from build123d import *

# Parameters (mm, degrees)
BOSS_EXTRUDE1_DEPTH          = 41.656
CUT_EXTRUDE1_DEPTH           = 38.481
CUT_EXTRUDE2_START           = -28.8671
SKETCH11_W                   = 16.434556017
SKETCH11_H                   = 15.968225366
CUT_EXTRUDE2_DEPTH           = 7.62
SKETCH16_W                   = 24.568216569
SKETCH16_H                   = 19.806256701
BOSS_EXTRUDE3_DEPTH          = 53.34
CUT_EXTRUDE3_START           = -24.568216569
CUT_EXTRUDE3_DEPTH           = 24.568216569
SKETCH22_W                   = 16.862412739
SKETCH22_H                   = 15.968225366
CUT_EXTRUDE4_DEPTH           = 53.34
CUT_EXTRUDE6_DEPTH           = 119.901499034
F_10_0_1935_DIAMETER_HOLE1_D = 4.9149
CUT_EXTRUDE11_REACH          = 116.77
CUT_EXTRUDE9_DEPTH           = 112.875933154
FILLET2_R                    = 2.54
SKETCH34_W                   = 28.194
SKETCH34_H                   = 38.481
BOSS_EXTRUDE4_DEPTH          = 3.302


# Read off the part's stored shape, not the designer's step: Cut-Extrude3
with BuildPart() as part:
    # Sketch1 → Boss-Extrude1 (new body)
    with BuildSketch(Plane(origin=(0, 0, 0), x_dir=(1, 0, 0), z_dir=(0, 1, 0))):
        with BuildLine():
            Line((63.017839503, -66.782093), (53.468205472, -26.506342671))
            Line((53.468205472, -26.506342671), (-35.875703335, -47.690346072))
            Line((-35.875703335, -47.690346072), (-26.326069304, -87.966096401))
            ThreePointArc((-26.326069304, -87.966096401), (21.184003401, -89.343908807), (63.017839503, -66.782093))
        make_face()
    extrude(amount=BOSS_EXTRUDE1_DEPTH)

    # Sketch2 → Cut-Extrude1 (cut)
    with BuildSketch(Plane(origin=(0, 41.656, 0), x_dir=(1, 0, 0), z_dir=(0, 1, 0))):
        Polygon((19.413866358, -81.878324539), (52.259801297, -74.090346526), (45.755169548, -46.656947141), (-3.674378893, -58.377004348), (2.830252857, -85.810403732), align=None)
    extrude(amount=-CUT_EXTRUDE1_DEPTH, mode=Mode.SUBTRACT)

    # Sketch11 → Cut-Extrude2 (cut)
    with BuildSketch(Plane(origin=(-44.671954403, 0, 10.592001701), x_dir=(0.230709787533386, 0, 0.973022607104429), z_dir=(-0.973022607104429, 0, 0.230709787533386)).offset(CUT_EXTRUDE2_START)):
        with Locations((69.159923537, 24.869161711)):
            Rectangle(SKETCH11_W, SKETCH11_H)
    extrude(amount=CUT_EXTRUDE2_DEPTH, mode=Mode.SUBTRACT)

    # Sketch16 → Boss-Extrude3 (add)
    with BuildSketch(Plane(origin=(-33.786311583, 0, 16.678693854), x_dir=(0, -1, 0), z_dir=(0.8966923373350206, 0, -0.4426543258171746))):
        with Locations((-23.482416275, -61.32247831)):
            Rectangle(SKETCH16_W, SKETCH16_H)
    extrude(amount=-BOSS_EXTRUDE3_DEPTH)

    # Cut-Extrude3 outline → Cut-Extrude3 (cut)
    with BuildSketch(Plane(origin=(0, 35.766524559, 0), x_dir=(1, 0, 0), z_dir=(0, 1, 0)).offset(CUT_EXTRUDE3_START)):
        with BuildLine():
            Line((-50.087557959, -104.157331307), (-20.43350094, -89.518534843))
            ThreePointArc((-20.43350094, -89.518534843), (-33.301223909, -85.569413503), (-45.453344654, -79.781511021))
            Line((-45.453344654, -79.781511021), (-58.854883166, -86.397212692))
            Line((-58.854883166, -86.397212692), (-50.087557959, -104.157331307))
        make_face()
    extrude(amount=CUT_EXTRUDE3_DEPTH, mode=Mode.SUBTRACT)

    # Sketch22 → Cut-Extrude4 (cut)
    with BuildSketch(Plane(origin=(-33.786311583, 0, 16.678693854), x_dir=(-0.4426543258171747, 0, -0.8966923373350206), z_dir=(0.8966923373350207, 0, -0.44265432581717473))):
        with Locations((-62.30694919, 24.869161711)):
            Rectangle(SKETCH22_W, SKETCH22_H)
    extrude(amount=-CUT_EXTRUDE4_DEPTH, mode=Mode.SUBTRACT)

    # Sketch24 → Cut-Extrude6 (cut, through all)
    with BuildSketch(Plane(origin=(0, 41.656, 0), x_dir=(1, 0, 0), z_dir=(0, 1, 0))):
        Polygon((56.919592876, -82.490265238), (45.99293133, -36.406877021), (-47.298720085, -58.526915055), (-50.529685657, -44.900260642), (55.061086644, -19.864023596), (69.218713762, -79.574066225), align=None)
    extrude(amount=-CUT_EXTRUDE6_DEPTH, mode=Mode.SUBTRACT)

    # #10 (0.1935) Diameter Hole1 (through all)
    with Locations(Plane(origin=(0, 41.656, 0), x_dir=(1, 0, 0), z_dir=(0, 1, 0))):
        with Locations((-9.275051774, -54.705205641), (35.043117703, -45.428524284)):
            Hole(F_10_0_1935_DIAMETER_HOLE1_D / 2)

    # Cut-Extrude11: up to this face of the body (flat: up to its plane)
    cut_extrude11_end = Plane(part.part.faces().sort_by_distance((24.292711202, 3.175, 66.233675437))[0])
    # Sketch33 → Cut-Extrude11 (cut, up to the picked face)
    with BuildSketch(Plane(origin=(0, 41.656, 0), x_dir=(1, 0, 0), z_dir=(0, 1, 0)), mode=Mode.PRIVATE) as cut_extrude11_sk1:
        Polygon((-6.887299542, -59.138808066), (13.024531054, -54.417587641), (19.529162804, -81.850987026), (-0.382667792, -86.572207451), align=None)
    cut_extrude11_tool1 = split(extrude(cut_extrude11_sk1.sketch, amount=-CUT_EXTRUDE11_REACH, mode=Mode.PRIVATE), bisect_by=cut_extrude11_end, keep=Keep.BOTH, mode=Mode.PRIVATE)
    add(cut_extrude11_tool1.solids().sort_by(Axis((6.320932, 41.656, 70.494898), (0, -1, 0)))[0], mode=Mode.SUBTRACT)

    # Sketch30 → Cut-Extrude9 (cut, through all)
    with BuildSketch(Plane.XZ.offset(-32.853274394)):
        Polygon((-5.736469349, 63.992454746), (-1.944856422, 79.983649289), (-5.130071965, 80.738883952), (-8.921684892, 64.74768941), align=None)
    extrude(amount=-CUT_EXTRUDE9_DEPTH, mode=Mode.SUBTRACT)

    # Fillet2
    fillet2_edges = [part.edges().sort_by_distance(p)[0] for p in [
        (-34.051060037, 20.828, 55.385811433),
        (45.99293133, 20.828, 36.406877021),
        (-37.760453577, 11.19830799, 75.983896866),
        (-37.760453577, 35.766524559, 75.983896866),
    ]]
    fillet(fillet2_edges, radius=FILLET2_R)

    # Sketch34 → Boss-Extrude4 (add)
    with BuildSketch(Plane(origin=(32.845934939, 0, -7.787978014), x_dir=(0.23070978753338592, 0, 0.973022607104429), z_dir=(-0.9730226071044291, 0, 0.23070978753338595))):
        with Locations((70.051429791, 22.4155)):
            Rectangle(SKETCH34_W, SKETCH34_H)
    extrude(amount=BOSS_EXTRUDE4_DEPTH)


solid = part.part
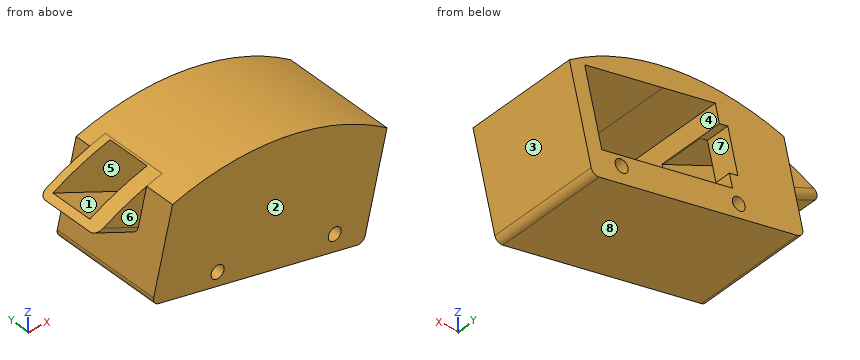
Here's how the part is built. I have some questions about the finished solid (model axes, mm). Face numbers are marked on the shaded views. A direction names the side the tool comes from. Round coordinates to 2 decimals unless told otherwise and drop trailing zeros. Order: outer loops, then holes, each group sorted by start corner. A loop starts at its lowest first (then second) coordinate and runs counter-clockwise, first axis right, second up. Notation, with made-up numbers: M 89.5,-14 L 140.5,-14 A9 ccw 140.5,-1 Z; hole C 87,-28 d11. An arc over 180 degrees is marked long. Return JSON: item names as keys, results as strings. Group by question number.
1. If we section it at B-B on x = 39: List the corners of the cut face in (y, z) for me (3 decimals), then the cut area to 3 significant figures.
2. If we section it at D-D on z = 61.5: List the corners of the cut face in (x, y) for me (3 decimals), then the cut area to 3 significant figures.
3. Please list where these lines run through material, in increasing order: probe 1 along Y at (x, z) = (-16, 73.5); probe 2 along Z at (x, y) = (15, 18); probe 3 along Y at (x, z) = (-2.5, 67.5) (3 decimals).
4. If we section it at A-A on y = 8.5: List the corners of the cut face in (x, z) for me, then the cut area to 3 significant figures.
5. If we section it at C-C on y = 19.5: List the corners of the cut face in (x, z) for me.
6. If we mould it in two halves opening along Z, with no side actions, what happens to the marked faces 1, 2, 3 and 4? For each: pulls with the +Z half, pulls with the -Z half, needs draft (parallel to the pull), parting line crosses it, or undercut.
7. On a 3-axis mill with a long thin cutter (end or side, diameter ignored), from which of +Z, -Z, +X, -X, +Y, -Y can I reach the whole of each face in a straight line? I mean the marked faces 5, 6, 7 and 8. Say none if no direction works.
8. I'm going to push flat-ended pins straight in: pin 1 Ø5 at (x, y) = (-32, 27.5) entering from +Z; pin 2 Ø8 at (y, z) = (13, 73) entering from -X; pin 3 Ø19.5 at (x, z) = (12, 67) entering from +Y (3 decimals). Where does each tip first touch, or does it pass through?
Reply:
{
 "1": {"outline": "M 0,38.065 L 41.656,38.065 L 41.656,48.259 L 3.175,48.259 L 3.175,77.234 L 41.656,77.234 L 41.656,83.127 L 0,83.127 Z", "area": "762 mm^2"},
 "2": {"outline": "M -32.601,0 L 51.943,0 L 51.943,41.656 L 45.881,41.656 L 45.881,3.175 L -6.327,3.175 L -6.327,41.656 L -32.601,41.656 Z", "area": "1,510 mm^2"},
 "3": {"probe 1": "0 to 16.89, 32.85 to 41.66", "probe 2": "43.76 to 53.95, 82.92 to 90.59", "probe 3": "0 to 3.175"},
 "4": {"outline": "M -33.47,57.86 A2.54 ccw -31.58,54.8 L 43.52,36.99 A2.54 ccw 46.58,38.88 L 54.83,73.66 A91.82 ccw -26.33,87.97 Z; hole C -9.28,54.71 d4.91; hole M -6.89,59.14 L 42.54,47.42 L 49.05,74.85 L -0.38,86.57 Z; hole C 35.04,45.43 d4.91", "area": "2,020 mm^2"},
 "5": {"outline": "M -45.45,79.78 L -30.07,72.19 L -33.47,57.86 A2.54 ccw -31.58,54.8 L 43.52,36.99 A2.54 ccw 46.58,38.88 L 54.83,73.66 A91.82 ccw -21.18,89.34 L -2.47,80.11 L -1.94,79.98 L -0.38,86.57 L 49.05,74.85 L 42.54,47.42 L -6.89,59.14 L -5.74,63.99 L -9.94,64.99 L -42.82,81.22 A91.82 ccw Z; hole C -9.28,54.71 d4.91; hole C 35.04,45.43 d4.91"},
 "6": {"face 1": "undercut", "face 2": "needs draft", "face 3": "pulls with the -Z half", "face 4": "undercut"},
 "7": {"face 5": "none", "face 6": "+Z, -X, -Y", "face 7": "+Y", "face 8": "-Z, -X, +Y, -Y"},
 "8": {"pin 1": "z = 77.11", "pin 2": "x = -39.73", "pin 3": "y = 3.175"}
}
